Could you check a few things on this drawing? It's one solid part, dimensions in mm from its lowest x, y, z. A direction names the side the tool comes from. Give positions to 0.01 mm unless a question says otherwise; leave off trailing zeros. Loops run counter-clockwise (first coordinate to the right, second up) from the corner with the lowest first, then second, coordinate; pieces in that order, holes last. Notation, with made-up numbers: M 54.5,65 L 79.5,65 A19 cw 79.5,91 Z; hole C -17.75,-6.5 d11. An arc over 180 degrees is marked long. Answer as CSV lines item,"result". Start each with the question number.
Item 1: For the marked faces 1, 2 and 3, which set-ups out of +Z, -Z, +X, -X, +Y, -Y let a thin tool reach every point of the face, with its end or its side?
Item 2: I want a section at A-A on y = 33. List the corners of the cut face in (x, z) for me, plus the area to 3 significant figures.
Item 3: Will these pins go through, and if not, where does the flat tip stop? P1, Ø5, axis at x = 23, z = 20.5, coming from the +Y side; P2, Ø8, axis at x = 73.5, y = 40.5, coming from the -Z side; P3, Ø23.5, axis at y = 33, z = 20, coming from the +X side; P4, Ø9, axis at x = 44.5, z = 20, coming from the +Y side.
Item 4: I want a section at C-C on x = 44.5. List the corners of the cut face in (y, z) for me.
Item 5: I want a section at D-D on z = 20. Give the number of separate pieces and of enclosed holes in the cut face, plus the area to 4 significant figures.
Item 6: If I drill on line 1 along Z through (x, y) = (44.5, 60.5); line 2 along Z through (x, y) = (65, 33); line 3 along Y through (x, z) = (79, 20), over which ranges is the centre line in solid material (lowest first)? Write a range as from..to.
Item 7: If we mould it in two halves opening along Z, with no side actions, what happens to the marked faces 4, 5 and 6? For each: released by +Z, released by -Z, zero draft, split by the parting line, or undercut.
Item 8: I want a section at B-B on x = 53.5. List the corners of the cut face in (y, z) for me, plus the area to 3 significant figures.
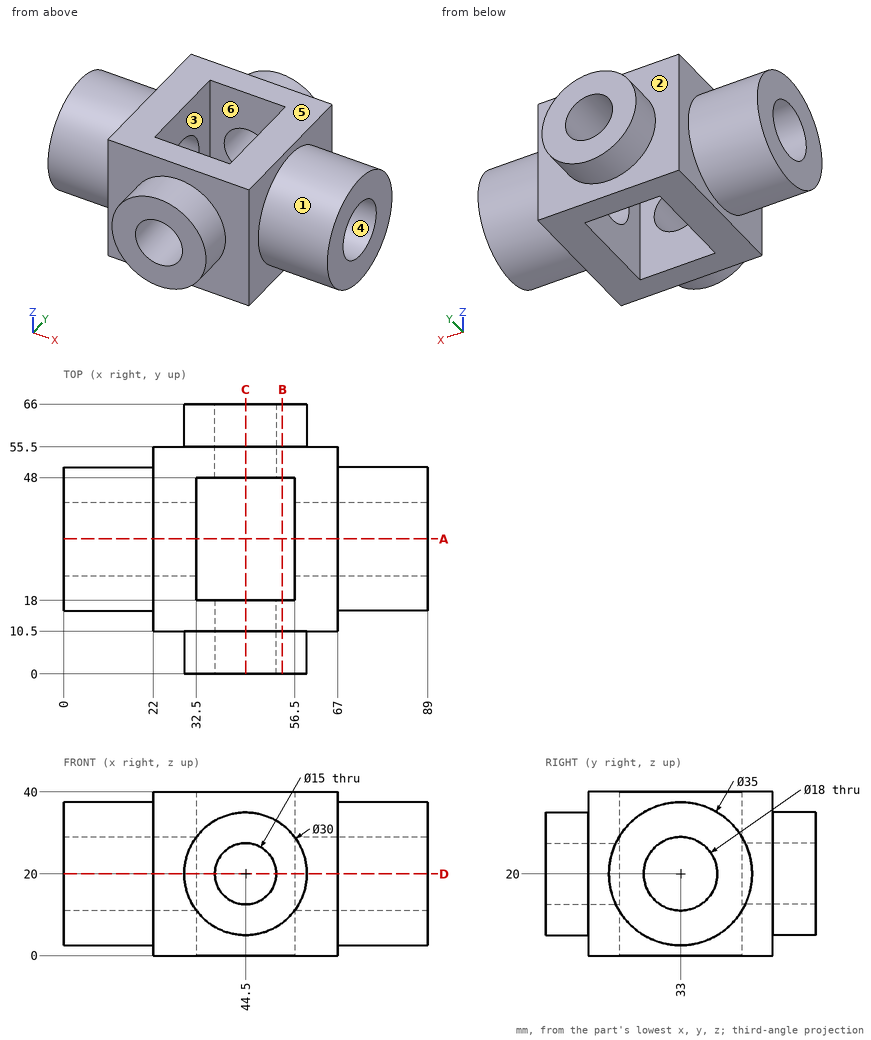
Result:
1,face 1,"+X"
1,face 2,"+Y"
1,face 3,"+Z, -Z"
2,outline,"M 0,2.5 L 22,2.5 L 22,0 L 32.5,0 L 32.5,11 L 0,11 Z; M 0,29 L 32.5,29 L 32.5,40 L 22,40 L 22,37.5 L 0,37.5 Z; M 56.5,0 L 67,0 L 67,2.5 L 89,2.5 L 89,11 L 56.5,11 Z; M 56.5,29 L 89,29 L 89,37.5 L 67,37.5 L 67,40 L 56.5,40 Z"
2,area,"1,210 mm^2"
3,P1,"y = 55.5"
3,P2,"z = 2.85"
3,P3,"x = 89"
3,P4,"through"
4,outline,"M 0,5 L 10.5,5 L 10.5,0 L 18,0 L 18,12.5 L 0,12.5 Z; M 0,27.5 L 18,27.5 L 18,40 L 10.5,40 L 10.5,35 L 0,35 Z; M 48,0 L 55.5,0 L 55.5,5 L 66,5 L 66,12.5 L 48,12.5 Z; M 48,27.5 L 66,27.5 L 66,35 L 55.5,35 L 55.5,40 L 48,40 Z"
5,separate pieces,"4"
5,enclosed holes,"0"
5,area,"1,765 mm^2"
6,line 1,"5..12.5, 27.5..35"
6,line 2,"0..11, 29..40"
6,line 3,"15.5..24, 42..50.5"
7,face 4,"undercut"
7,face 5,"released by +Z"
7,face 6,"zero draft"
8,outline,"M 0,8 L 10.5,8 L 10.5,0 L 18,0 L 18,40 L 10.5,40 L 10.5,32 L 0,32 Z; M 48,0 L 55.5,0 L 55.5,8 L 66,8 L 66,32 L 55.5,32 L 55.5,40 L 48,40 Z"
8,area,"1,100 mm^2"
